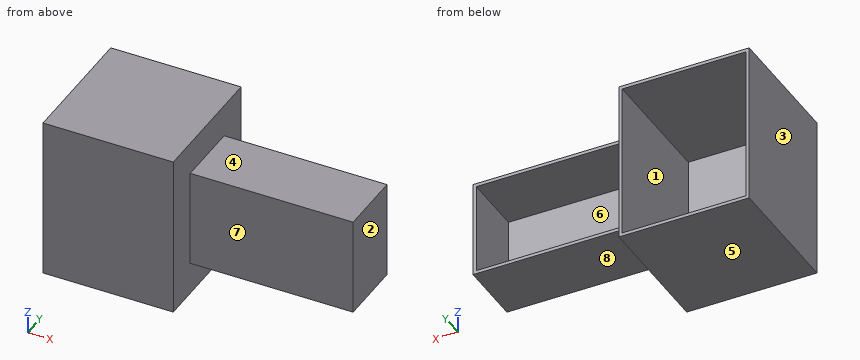
```python
from build123d import *

# Parameters (mm, degrees)
SKETCH1_W           = 101.6
SKETCH1_H           = 127
SKETCH1_W_2         = 96.52
SKETCH1_H_2         = 121.92
EXTRUDE_THIN1_DEPTH = 101.6
SKETCH1_2_W         = 101.6
SKETCH1_2_H         = 127
BOSS_EXTRUDE1_DEPTH = 2.54
SKETCH2_W           = 127
SKETCH2_H           = 76.2
SKETCH2_W_2         = 121.92
SKETCH2_H_2         = 71.12
EXTRUDE_THIN2_DEPTH = 50.8
SKETCH2_2_W         = 127
SKETCH2_2_H         = 76.2
BOSS_EXTRUDE2_DEPTH = 2.54


with BuildPart() as part:
    # Sketch1 → Extrude-Thin1 (new body)
    with BuildSketch(Plane(origin=(0, 0, 0), x_dir=(1, 0, 0), z_dir=(0, 1, 0))):
        Rectangle(SKETCH1_W, SKETCH1_H)
        Rectangle(SKETCH1_W_2, SKETCH1_H_2, mode=Mode.SUBTRACT)
    extrude(amount=EXTRUDE_THIN1_DEPTH)

    # Sketch1<2> → Boss-Extrude1 (add)
    with BuildSketch(Plane(origin=(0, 0, 0), x_dir=(1, 0, 0), z_dir=(0, 1, 0))):
        Rectangle(SKETCH1_2_W, SKETCH1_2_H)
    extrude(amount=BOSS_EXTRUDE1_DEPTH)

    # Sketch2 → Extrude-Thin2 (add)
    with BuildSketch(Plane(origin=(0, 25.4, 0), x_dir=(1, 0, 0), z_dir=(0, 1, 0))):
        with Locations((114.3, 0)):
            Rectangle(SKETCH2_W, SKETCH2_H)
        with Locations((114.3, 0)):
            Rectangle(SKETCH2_W_2, SKETCH2_H_2, mode=Mode.SUBTRACT)
    extrude(amount=EXTRUDE_THIN2_DEPTH)

    # Sketch2<2> → Boss-Extrude2 (add)
    with BuildSketch(Plane(origin=(0, 25.4, 0), x_dir=(1, 0, 0), z_dir=(0, 1, 0))):
        with Locations((114.3, 0)):
            Rectangle(SKETCH2_2_W, SKETCH2_2_H)
    extrude(amount=BOSS_EXTRUDE2_DEPTH)


solid = part.part
```
Could you check a few things on this model? Use its own coordinates, in mm. Face numbers are marked on the shaded views. A direction names the side the tool comes from. Round coordinates to 2 decimals unless told otherwise and drop trailing zeros. Write each loop counter-clockwise with the first axis right and the second up, starting at its lowest first coordinate (ties: lowest second). Pieces come first, ordered by that corner, then holes.
(1) Thinking about a two-plate mould opening in X: for the marked faces 1, 2, 3 and 4, which applies, +X half, -X half, draft (parallel to the pull), parting line (faces both ways), or undercut?
Findings below:
face 1: undercut
face 2: +X half
face 3: -X half
face 4: draft
(2) If I drill on probe 1 along X at (y, z) = (62, 8); probe 2 along Z at (x, y) = (-20, 35); probe 3 along X at (y, z) = (80, -24), over which ranges is the centre line in solid material (lowest first)?
Findings below:
probe 1: x = -50.8 to -48.26, 48.26 to 53.34, 175.26 to 177.8
probe 2: z = -63.5 to -60.96, 60.96 to 63.5
probe 3: x = -50.8 to -48.26, 48.26 to 50.8
(3) Suppose I cut it at C-C on y = 14. Write out the boundary of the cut face in (x, z), and give its area (3 significant figures).
Findings below:
outline: (-50.8, -63.5) - (50.8, -63.5) - (50.8, 63.5) - (-50.8, 63.5) - close; hole (-48.26, -60.96) - (48.26, -60.96) - (48.26, 60.96) - (-48.26, 60.96) - close
area: 1,140 mm2
(4) Which directions (+Z, -Z, +X, -X, +Y, -Y) give clear straight access to the entire face, cutting with the end or side of a thin tool? Please do the marked faces 5, 6, 7 and 8.
Findings below:
face 5: -Z, +X, -X, +Y, -Y
face 6: +Y
face 7: +Z, -Z, +X, -Y
face 8: -Z, +X, +Y, -Y
(5) Suppose I cut it at A-A on x = 98. Write out the boundary of the cut face in (y, z), and give its area (3 significant figures).
Findings below:
outline: (25.4, -38.1) - (76.2, -38.1) - (76.2, -35.56) - (27.94, -35.56) - (27.94, 35.56) - (76.2, 35.56) - (76.2, 38.1) - (25.4, 38.1) - close
area: 439 mm2
(6) Suppose I cut it at D-D on z = -46.5. Write out the boundary of the cut face in (x, y).
Findings below:
outline: (-50.8, 0) - (50.8, 0) - (50.8, 101.6) - (48.26, 101.6) - (48.26, 2.54) - (-48.26, 2.54) - (-48.26, 101.6) - (-50.8, 101.6) - close
(7) For pin 1 (6 mm diameter, centred on x = 76.5, z = -29, fed in from -Y); pin 2 (24 mm diameter, centred on x = 84.5, y = 53.5, fed in from +Z); pin 3 (1.5 mm diameter, centred on x = 111.5, y = 71.5, fed in from -Z), each with a flat end and sliding along its axis, tell me the tip position at first contact or that it passes through.
Findings below:
pin 1: stops at y = 25.4
pin 2: stops at z = 38.1
pin 3: stops at z = -38.1
(8) Suppose I cut it at B-B on y = 39. Write out the boundary of the cut face in (x, z), and give its area (3 significant figures).
Findings below:
outline: (-50.8, -63.5) - (50.8, -63.5) - (50.8, -38.1) - (177.8, -38.1) - (177.8, 38.1) - (50.8, 38.1) - (50.8, 63.5) - (-50.8, 63.5) - close; hole (-48.26, -60.96) - (48.26, -60.96) - (48.26, 60.96) - (-48.26, 60.96) - close; hole (53.34, -35.56) - (175.26, -35.56) - (175.26, 35.56) - (53.34, 35.56) - close
area: 2,140 mm2
